Read the model definition and answer for the solid it produces. Units are mm, in the model's axes. A direction names the side the tool comes from. Coordinates: 2 decimals unless noted, no trailing zeros. Write each loop counter-clockwise with the first axis right and the second up, starting at its lowest first coordinate (ties: lowest second). Pieces come first, ordered by that corner, then holes. Notation, with made-up numbers: (66.5, -32.5) -> (91.5, -32.5) arc R22 cw to (91.5, -16.5) -> close; hole circle Ø8 at (24.25, -17.75). An arc over 180 degrees is marked (long way). Write item = value, one per line. Start each with the question number.
1) Find the intervals of material crossed by line 1 along X through (y, z) = (-2.25, 1.05); line 2 along Y through (x, z) = (2.75, -1.8); line 3 along Z through (x, y) = (1, -1.9), in increasing order. Write a range as from..to.
2) A tool of negligible diameter and unlimited length cuts with its end or side. For faces 1 (the face through (0, 1.1, -1.1)), 2 (the face through (3, 0, 2)), 3 (the face through (1, 0, -1.26)), from which of +Z, -Z, +X, -X, +Y, -Y can it reach the whole face along a straight path? Write none if from no direction.
3) A flat-ended cylindrical pin translates along its axis: pin 1 Ø1.5 at (x, y) = (7.5, 0.5) entering from +Z. Find the tip coordinate at first contact, or state that the pin passes through.
4) Section A-A (x = 1.5) is taken. Determine the outline of the cut face in (y, z).
from build123d import *

# Parameters (mm, degrees)
FILLET1_R       = 0.1
FILLET2_R       = 0.3
HEX_2_DEPTH     = 1.3
THDSCHPAT_COUNT = 9
THDSCHPAT_PITCH = 0.5


with BuildPart() as part:
    # BodySke → Base-Revolve (revolve)
    with BuildSketch(Plane.XY, mode=Mode.PRIVATE) as base_revolve_sk:
        Polygon((0, 0), (0, 2.75), (3, 2.75), (3, 1.5), (8.7195, 1.5), (9, 1.2195), (9, 0), align=None)
    revolve(base_revolve_sk.sketch.rotate(Axis((-31.75, 0, 0), (1, 0, 0)), 90), axis=Axis((-31.75, 0, 0), (1, 0, 0)))

    # Fillet1
    fillet1_edges = [part.edges().sort_by_distance(p)[0] for p in [
        (3, 0, -1.5),
    ]]
    fillet(fillet1_edges, radius=FILLET1_R)

    # Fillet2
    fillet2_edges = [part.edges().sort_by_distance(p)[0] for p in [
        (0, 0, -2.75),
    ]]
    fillet(fillet2_edges, radius=FILLET2_R)

    # Sketch2 → Hex-PreBroach (revolve, cut)
    with BuildSketch(Plane.XY, mode=Mode.PRIVATE) as hex_prebroach_sk:
        Polygon((0, 1.26), (1.3, 1.26), (2.027461339, 0), (0, 0), align=None)
    revolve(hex_prebroach_sk.sketch.rotate(Axis((0, 0, 0), (1, 0, 0)), 90), axis=Axis((0, 0, 0), (1, 0, 0)), mode=Mode.SUBTRACT)

    # Sketch3 → Hex 2 (cut)
    with BuildSketch(Plane(origin=(0, 0, 0), x_dir=(0, 0.500000000000001, 0.866025403784438), z_dir=(-1, 0, 0))):
        Polygon((0.727461339, 1.26), (-0.727461339, 1.26), (-1.454922678, 0), (-0.727461339, -1.26), (0.727461339, -1.26), (1.454922678, 0), align=None)
    extrude(amount=-HEX_2_DEPTH, mode=Mode.SUBTRACT)

    # ThdSchSke → ThreadSchematic (revolve, cut)
    with BuildSketch(Plane.XY):
        Polygon((4.5, -1.2195), (4.303591786, -1.5), (4.303591786, -1.875), (4.696408214, -1.875), (4.696408214, -1.5), align=None)
    threadschematic = revolve(axis=Axis((-3.175, 0, 0), (1, 0, 0)), mode=Mode.SUBTRACT)

    # ThdSchPat: ThreadSchematic ×9
    with Locations(*[(i * THDSCHPAT_PITCH, 0, 0) for i in range(1, THDSCHPAT_COUNT)]):
        add(threadschematic, mode=Mode.SUBTRACT)


solid = part.part
Answer key:
q1.line_1 = 0..3
q1.line_2 = -2.08..2.08
q1.line_3 = -1.99..1.99
q2.face_1 = +Z, -Z, -X, +Y, -Y
q2.face_2 = +X
q2.face_3 = -X
q3.pin_1 = 1.5
q4.outline = circle Ø5.5 at (0, 0); hole circle Ø1.83 at (0, 0)
